The model under review builds one solid part; all positions refer to its coordinate system, in mm. Coordinates: 2 decimals unless noted, no trailing zeros. Write each loop counter-clockwise with the first axis right and the second up, starting at its lowest first coordinate (ties: lowest second). Pieces come first, ordered by that corner, then holes. Notation, with made-up numbers: (2, 81) - (30, 81) arc R4 ccw to (30, 85) - close; hole circle Ø10 at (11.5, 25.5). An arc over 180 degrees is marked (long way). Put each result on its own line as item: value.
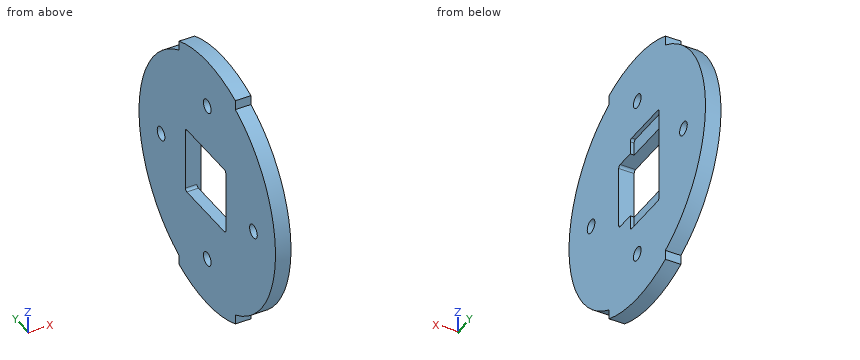
from build123d import *

# Parameters (mm, degrees)
BOSS_EXTRUDE1_DEPTH      = 6
CUT_EXTRUDE1_DEPTH       = 20
M5_CLEARANCE_HOLE1_D     = 5.3
M5_CLEARANCE_HOLE1_DEPTH = 15
M5_CLEARANCE_HOLE1_TIP   = 1.59228064
CUT_EXTRUDE2_DEPTH       = 1.5
FILLET1_R                = 1


with BuildPart() as part:
    # Sketch1 → Boss-Extrude1 (new body)
    with BuildSketch(Plane(origin=(0, 0, 0), x_dir=(0, 0, -1), z_dir=(1, 0, 0))):
        with BuildLine():
            Line((-46.8, 19.5), (-43.038500206, 19.5))
            ThreePointArc((-43.038500206, 19.5), (0, 47.25), (43.038500206, 19.5))
            Line((43.038500206, 19.5), (46.8, 19.5))
            ThreePointArc((46.8, 19.5), (50.7, 0), (46.8, -19.5))
            Line((46.8, -19.5), (43.038500206, -19.5))
            ThreePointArc((43.038500206, -19.5), (0, -47.25), (-43.038500206, -19.5))
            Line((-43.038500206, -19.5), (-46.8, -19.5))
            ThreePointArc((-46.8, -19.5), (-50.7, 0), (-46.8, 19.5))
        make_face()
    extrude(amount=BOSS_EXTRUDE1_DEPTH)

    # Sketch2 → Cut-Extrude1 (cut)
    with BuildSketch(Plane(origin=(6, 0, 0), x_dir=(0, 0, -1), z_dir=(1, 0, 0))):
        with BuildLine():
            ThreePointArc((12, -11.85), (12.707106781, -11.557106781), (13, -10.85))
            Line((13, -10.85), (13, -3.85))
            Line((13, -3.85), (13, 14.15))
            ThreePointArc((13, 14.15), (12.707106781, 14.857106781), (12, 15.15))
            Line((12, 15.15), (-12, 15.15))
            ThreePointArc((-12, 15.15), (-12.707106781, 14.857106781), (-13, 14.15))
            Line((-13, 14.15), (-13, -3.85))
            Line((-13, -3.85), (-13, -10.85))
            ThreePointArc((-13, -10.85), (-12.707106781, -11.557106781), (-12, -11.85))
            Line((-12, -11.85), (12, -11.85))
        make_face()
        with BuildLine():
            Line((-12, -12.85), (12, -12.85))
            ThreePointArc((12, -12.85), (12.707106781, -12.557106781), (13, -11.85))
            Line((13, -11.85), (13, -10.85))
            ThreePointArc((13, -10.85), (12.707106781, -11.557106781), (12, -11.85))
            Line((12, -11.85), (-12, -11.85))
            ThreePointArc((-12, -11.85), (-12.707106781, -11.557106781), (-13, -10.85))
            Line((-13, -10.85), (-13, -11.85))
            ThreePointArc((-13, -11.85), (-12.707106781, -12.557106781), (-12, -12.85))
        make_face()
    extrude(amount=-CUT_EXTRUDE1_DEPTH, mode=Mode.SUBTRACT)

    # M5 Clearance Hole1
    with Locations(Plane.ZY):
        with Locations((-32, 0), (0, 32), (32, 0), (0, -32)):
            Hole(M5_CLEARANCE_HOLE1_D / 2, depth=M5_CLEARANCE_HOLE1_DEPTH)
            with Locations((0, 0, -(M5_CLEARANCE_HOLE1_DEPTH + M5_CLEARANCE_HOLE1_TIP / 2))):  # 118° drill point
                Cone(0, M5_CLEARANCE_HOLE1_D / 2, M5_CLEARANCE_HOLE1_TIP, mode=Mode.SUBTRACT)

    # Sketch16 → Cut-Extrude2 (cut)
    with BuildSketch(Plane(origin=(6, 0, 0), x_dir=(0, 0, -1), z_dir=(1, 0, 0))):
        with BuildLine():
            ThreePointArc((-13, 14.15), (-12.707106781, 14.857106781), (-12, 15.15))
            Line((-12, 15.15), (-19, 15.15))
            Line((-19, 15.15), (-19, -4.85))
            Line((-19, -4.85), (-13, -4.85))
            Line((-13, -4.85), (-13, 14.15))
        make_face()
        with BuildLine():
            Line((0, -4.85), (0, 15.15))
            Line((0, 15.15), (-12, 15.15))
            ThreePointArc((-12, 15.15), (-12.707106781, 14.857106781), (-13, 14.15))
            Line((-13, 14.15), (-13, -4.85))
            Line((-13, -4.85), (0, -4.85))
        make_face()
        with BuildLine():
            ThreePointArc((13, 14.15), (12.707106781, 14.857106781), (12, 15.15))
            Line((12, 15.15), (0, 15.15))
            Line((0, 15.15), (0, -4.85))
            Line((0, -4.85), (13, -4.85))
            Line((13, -4.85), (13, 14.15))
        make_face()
        with BuildLine():
            Line((19, -4.85), (19, 15.15))
            Line((19, 15.15), (12, 15.15))
            ThreePointArc((12, 15.15), (12.707106781, 14.857106781), (13, 14.15))
            Line((13, 14.15), (13, -4.85))
            Line((13, -4.85), (19, -4.85))
        make_face()
    extrude(amount=-CUT_EXTRUDE2_DEPTH, mode=Mode.SUBTRACT)

    # Fillet1
    fillet1_edges = [part.edges().sort_by_distance(p)[0] for p in [
        (5.25, 15.15, 19),
        (5.25, -4.85, -19),
        (5.25, -4.85, 19),
        (5.25, 15.15, -19),
    ]]
    fillet(fillet1_edges, radius=FILLET1_R)


solid = part.part
1. Consider section B-B on x = 3.15. State the section outline as (y, z) points, plus the area to 3 significant figures.
Determined:
outline: (-19.5, -46.8) arc R50.7 ccw to (19.5, -46.8) - (19.5, -43.04) arc R47.25 ccw to (19.5, 43.04) - (19.5, 46.8) arc R50.7 ccw to (-19.5, 46.8) - (-19.5, 43.04) arc R47.25 ccw to (-19.5, -43.04) - close; hole circle Ø5.3 at (-32, 0); hole (-12.85, -12) arc R1 ccw to (-11.85, -13) - (14.15, -13) arc R1 ccw to (15.15, -12) - (15.15, 12) arc R1 ccw to (14.15, 13) - (-11.85, 13) arc R1 ccw to (-12.85, 12) - close; hole circle Ø5.3 at (0, -32); hole circle Ø5.3 at (0, 32); hole circle Ø5.3 at (32, 0)
area: 6,480 mm^2
2. Consider section A-A on y = 0. State the section outline as (x, z) points.
Determined:
outline: (0, -50.7) - (6, -50.7) - (6, -34.65) - (0, -34.65) - close; (0, -29.35) - (6, -29.35) - (6, -19) - (4.5, -19) - (4.5, -13) - (0, -13) - close; (0, 13) - (4.5, 13) - (4.5, 19) - (6, 19) - (6, 29.35) - (0, 29.35) - close; (0, 34.65) - (6, 34.65) - (6, 50.7) - (0, 50.7) - close
3. Consider section C-C on z = 32. State the section outline as (x, y) points.
Determined:
outline: (0, -34.76) - (6, -34.76) - (6, -2.65) - (0, -2.65) - close; (0, 2.65) - (6, 2.65) - (6, 34.76) - (0, 34.76) - close
4. For pin 1 Ø1.2 at (x, y) = (5.5, 6.5) entering from +Z; pin 2 Ø1.6 at (x, z) = (5, -16) entering from +Y; pin 3 Ø1.1 at (x, z) = (3.5, 45) entering from -Y, all flat-tipped, find the tip position at first contact; note any pin that passes through.
Determined:
pin 1: stops at z = 50.36
pin 2: stops at y = 44.74
pin 3: stops at y = -19.5
5. To check wall thickness, follow probe 1 along Y at (x, z) = (4.05, 0); probe 2 along Y at (x, z) = (0.7, -11); probe 3 along Y at (x, z) = (5.1, 7.5). State the ranges of each line that lie inside material, in increasing order.
Determined:
probe 1: y = -47.25 to -34.65, -29.35 to -12.85, 15.15 to 29.35, 34.65 to 47.25
probe 2: y = -45.95 to -12.85, 15.15 to 45.95
probe 3: y = -46.65 to -12.85, 15.15 to 46.65
